Here's how the part is built. I have some questions about the finished solid (model axes, mm). A direction names the side the tool comes from. Give positions to 0.01 mm unless a question says otherwise; leave off trailing zeros. Loops run counter-clockwise (first coordinate to the right, second up) from the corner with the lowest first, then second, coordinate; pieces in that order, holes last. Notation, with made-up numbers: (11.5, 40.25) -> (40.5, 40.25) arc R29 cw to (40.5, 71.25) -> close; hole circle Ø7 at (21.5, -6.75). An arc over 180 degrees is marked (long way). Answer in a Markdown table with one row per item. Add a question column.
Item 1: For P1, Ø3, axis at x = -70, y = 9, coming from the -Z side; P2, Ø1.8, axis at x = 52.5, z = 2.5, coming from the -Y side, each with a flat end and sliding along its axis, tell me the tip position at first contact or that it passes through.
Item 2: If we section it at B-B (x = 85.5): Write out the boundary of the cut face in (y, z), then the cut area to 3 significant figures.
Item 3: We'd pull the mould along X, two halves only. Please class faces 1 (the face through (-1.6, 15, 3)), 2 (the face through (110, -17, 3)): released by +X, released by -X, zero draft, split by the parting line, or undercut.
Item 4: Which directions (+Z, -Z, +X, -X, +Y, -Y) give clear straight access to the entire face, cutting with the end or side of a thin tool? Please do faces 3 (the face through (101.4, 15, 3)), 4 (the face through (15, -8, 3)), 5 (the face through (110, 17, 3)).
Item 5: If I drill on line 1 (X direction, y = -4, z = 5.3); line 2 (X direction, y = -9, z = 2.65); line 3 (X direction, y = 9.5, z = 0.5), over which ranges is the centre line in solid material (lowest first)?
Item 6: If we section it at A-A (z = 2.2): Give the number of separate pieces and of enclosed holes in the cut face, then the cut area to 3 significant figures.
```python
from build123d import *

# Parameters (mm, degrees)
ESBO_O1_R                = 1.6
RESSALTO_EXTRUS_O1_DEPTH = 6
ESBO_O2_R                = 1.6
ESBO_O2_W                = 75
ESBO_O2_H                = 18
CORTE_EXTRUS_O1_DEPTH    = 10


with BuildPart() as part:
    # Esboço1 → Ressalto-extrusão1 (new body)
    with BuildSketch(Plane.XY):
        Polygon((-115, 17), (-115, -17), (-104.6, -17), (-104.6, -13), (-106, -13), (-106, -10), (-104.6, -10), (-104.6, -7), (-101.4, -7), (-101.4, -10), (-100, -10), (-100, -13), (-101.4, -13), (-101.4, -17), (-1.6, -17), (-1.6, -13), (-3, -13), (-3, -10), (-1.6, -10), (-1.6, -7), (1.6, -7), (1.6, -10), (3, -10), (3, -13), (1.6, -13), (1.6, -17), (101.4, -17), (101.4, -13), (100, -13), (100, -10), (101.4, -10), (101.4, -7), (104.6, -7), (104.6, -10), (106, -10), (106, -13), (104.6, -13), (104.6, -17), (115, -17), (115, 17), (104.6, 17), (104.6, 13), (106, 13), (106, 10), (104.6, 10), (104.6, 7), (101.4, 7), (101.4, 10), (100, 10), (100, 13), (101.4, 13), (101.4, 17), (1.6, 17), (1.6, 13), (3, 13), (3, 10), (1.6, 10), (1.6, 7), (-1.6, 7), (-1.6, 10), (-3, 10), (-3, 13), (-1.6, 13), (-1.6, 17), (-101.4, 17), (-101.4, 13), (-100, 13), (-100, 10), (-101.4, 10), (-101.4, 7), (-104.6, 7), (-104.6, 10), (-106, 10), (-106, 13), (-104.6, 13), (-104.6, 17), align=None)
        with Locations((112, 0)):
            Circle(ESBO_O1_R, mode=Mode.SUBTRACT)
        Circle(ESBO_O1_R, mode=Mode.SUBTRACT)
        with Locations((-112, 0)):
            Circle(ESBO_O1_R, mode=Mode.SUBTRACT)
    extrude(amount=RESSALTO_EXTRUS_O1_DEPTH)

    # Esboço2 → Corte-extrusão1 (cut)
    with BuildSketch(Plane.XY.offset(6)):
        with Locations((70, 9)):
            Circle(ESBO_O2_R)
        with Locations((-70, 9)):
            Circle(ESBO_O2_R)
        with Locations((52.5, -8)):
            Rectangle(ESBO_O2_W, ESBO_O2_H)
        with Locations((-52.5, -8)):
            Rectangle(ESBO_O2_W, ESBO_O2_H)
    extrude(amount=-CORTE_EXTRUS_O1_DEPTH, mode=Mode.SUBTRACT)


solid = part.part
```
Recorded:
| question | item | result |
|---|---|---|
| 1 | P1 | passes through |
| 1 | P2 | stops at y = 1 |
| 2 | outline | (1, 0) -> (17, 0) -> (17, 6) -> (1, 6) -> close |
| 2 | area | 96.0 mm^2 |
| 3 | face 1 | undercut |
| 3 | face 2 | zero draft |
| 4 | face 3 | +Z, -Z, +Y |
| 4 | face 4 | +Z, -Z, -Y |
| 4 | face 5 | +Z, -Z, +X, -X, +Y |
| 5 | line 1 | x = -115 to -90, -15 to 15, 90 to 115 |
| 5 | line 2 | x = -115 to -104.6, -101.4 to -90, -15 to -1.6, 1.6 to 15, 90 to 101.4, 104.6 to 115 |
| 5 | line 3 | x = -115 to -104.6, -101.4 to -71.52, -68.48 to -1.6, 1.6 to 68.48, 71.52 to 101.4, 104.6 to 115 |
| 6 | separate pieces | 1 |
| 6 | enclosed holes | 5 |
| 6 | area | 4,840 mm^2 |
